from build123d import *

# Parameters (mm, degrees)
SKETCH1_R           = 10
BOSS_EXTRUDE1_DEPTH = 2
SKETCH2_R           = 4.5
BOSS_EXTRUDE2_DEPTH = 7
SKETCH3_R           = 1.275
CUT_EXTRUDE1_DEPTH  = 3
FILLET1_R           = 0.25
SKETCH6_R           = 1.15
CUT_EXTRUDE2_DEPTH  = 10
SKETCH7_R           = 3.25
CUT_EXTRUDE3_DEPTH  = 2.5
BOSS_EXTRUDE4_DEPTH = 2.5
CIRPATTERN1_COUNT   = 26


with BuildPart() as part:
    # Sketch1 → Boss-Extrude1 (new body)
    with BuildSketch(Plane(origin=(0, 0, 0), x_dir=(1, 0, 0), z_dir=(0, 1, 0))):
        Circle(SKETCH1_R)
    extrude(amount=BOSS_EXTRUDE1_DEPTH)

    # Sketch2 → Boss-Extrude2 (add)
    with BuildSketch(Plane(origin=(0, 0, 0), x_dir=(1, 0, 0), z_dir=(0, 1, 0))):
        Circle(SKETCH2_R)
    extrude(amount=-BOSS_EXTRUDE2_DEPTH)

    # Sketch3 → Cut-Extrude1 (cut, through all)
    with BuildSketch(Plane(origin=(0, 0, 0), x_dir=(1, 0, 0), z_dir=(0, 1, 0))):
        with Locations((0, 7)):
            Circle(SKETCH3_R)
        with Locations((-7, 0)):
            Circle(SKETCH3_R)
        with Locations((0, -7)):
            Circle(SKETCH3_R)
        with Locations((7, 0)):
            Circle(SKETCH3_R)
    extrude(amount=CUT_EXTRUDE1_DEPTH, mode=Mode.SUBTRACT)

    # Fillet1
    fillet1_edges = [part.edges().sort_by_distance(p)[0] for p in [
        (-10, 0, 0),
    ]]
    fillet(fillet1_edges, radius=FILLET1_R)

    # Sketch6 → Cut-Extrude2 (cut, through all)
    with BuildSketch(Plane(origin=(0, 2, 0), x_dir=(1, 0, 0), z_dir=(0, 1, 0))):
        Circle(SKETCH6_R)
    extrude(amount=-CUT_EXTRUDE2_DEPTH, mode=Mode.SUBTRACT)

    # Sketch7 → Cut-Extrude3 (cut)
    with BuildSketch(Plane.XZ.offset(7)):
        Circle(SKETCH7_R)
    extrude(amount=-CUT_EXTRUDE3_DEPTH, mode=Mode.SUBTRACT)

    # Sketch8 → Boss-Extrude4 (add)
    with BuildSketch(Plane.XZ.offset(7)):
        with BuildLine():
            Line((-2.67824125, -1.107011583), (-3.073819571, -1.003017967))
            ThreePointArc((-3.073819571, -1.003017967), (-2.972382473, -1.245868077), (-2.849346423, -1.478521878))
            Line((-2.849346423, -1.478521878), (-2.67824125, -1.107011583))
        make_face()
    boss_extrude4 = extrude(amount=-BOSS_EXTRUDE4_DEPTH)

    # CirPattern1: Boss-Extrude4 ×26 about axis
    cirpattern1_axis = Axis((0, 0, 0), (0, 1, 0))
    for i in range(1, CIRPATTERN1_COUNT):
        add(boss_extrude4.rotate(cirpattern1_axis, i * 360 / CIRPATTERN1_COUNT))


solid = part.part
Geometry: final body of the model. Coordinates: model frame, mm. A direction names the side the tool comes from. Give positions to 0.01 mm unless a question says otherwise; leave off trailing zeros. Write each loop counter-clockwise with the first axis right and the second up, starting at its lowest first coordinate (ties: lowest second). Pieces come first, ordered by that corner, then holes.
(1) First-contact query: P1, Ø3.5, axis at x = 0, z = 7, coming from the -Y side; P2, Ø4, axis at x = -7.5, y = 0.5, coming from the -Z side; P3, Ø2, axis at x = -1, z = 1, coming from the -Y side. Flat tips, straight axial feed; report the tip coordinate or a pass-through.
(2) Access query for faces 4 (the cylindrical face through (-8.274, 0.986, -0.056)), 5 (the cylindrical face through (-0.59, -3.45, -4.46)). Directions: +Z, -Z, +X, -X, +Y, -Y. A direction counts if a zero-diameter tool reaches every point of the face in a straight line with its end or side. Return the directions, or none.
(3) Ray query, line 1 (Z direction, x = 0, y = 1.45) (3 decimals); line 2 (Z direction, x = 0, y = -2.5). Return the intervals inside material, ascending.
(4) Cut plane A-A, the plane y = -0.75. Return loops of the section in (x, z), then the cut area to 3 significant figures.
(5) Mould query, pull axis X, two halves, no side actions, for faces 1 (the cylindrical face through (-2.17, 1.11, 9.76)), 2 (the cylindrical face through (5.726, 0.986, -0.056)), 3 (the flat face through (4.2, 0, 2)). Classes: released by +X, released by -X, zero draft, split by the parting line, or undercut.
Values follow:
1. P1: stops at y = 0
1. P2: stops at z = -8.35
1. P3: stops at y = -4.5
2. face 4: +Y, -Y
2. face 5: -Y
3. line 1: z = -10 to -8.275, -5.725 to -1.15, 1.15 to 5.725, 8.275 to 10
3. line 2: z = -4.5 to -1.15, 1.15 to 4.5
4. outline: circle Ø9 at (0, 0); hole circle Ø2.3 at (0, 0)
4. area: 59.5 mm2
5. face 1: split by the parting line
5. face 2: undercut
5. face 3: zero draft
